```python
from build123d import *

# Parameters (mm, degrees)
PAD007_DEPTH          = 0.8
PAD007_MIRROR_2_DEPTH = 0.8


with BuildPart() as part:
    # Sketch038 (on XZ_Plane013 of Origin026) → Pad007 (new body, symmetric)
    with BuildSketch(Plane.XZ):
        with BuildLine():
            Line((0, 6.3), (0, 0))
            Line((0, 0), (-8.5, 0))
            ThreePointArc((-8.5, 0), (-10, 1.5), (-11.5, 0))
            Line((-11.5, 0), (-12.5, 0))
            ThreePointArc((-10, 2.5), (-11.767767, 1.767767), (-12.5, 0))
            Line((-10, 2.5), (-7.85, 2.5))
            Line((-7.85, 2.5), (-7.85, 6.3))
            Line((-7.85, 6.3), (0, 6.3))
        make_face()
    pad007 = extrude(amount=PAD007_DEPTH, both=True)

    # Sketch038 Mirror 2 → Pad007 Mirror 2 (add, symmetric)
    with BuildSketch(Plane(origin=(0, 0, 0), x_dir=(-1, 0, 0), z_dir=(0, 1, 0))):
        with BuildLine():
            Line((0, 6.3), (0, 0))
            Line((0, 0), (-8.5, 0))
            ThreePointArc((-8.5, 0), (-10, 1.5), (-11.5, 0))
            Line((-11.5, 0), (-12.5, 0))
            ThreePointArc((-10, 2.5), (-11.767767, 1.767767), (-12.5, 0))
            Line((-10, 2.5), (-7.85, 2.5))
            Line((-7.85, 2.5), (-7.85, 6.3))
            Line((-7.85, 6.3), (0, 6.3))
        make_face()
    pad007_mirror_2 = extrude(amount=-PAD007_MIRROR_2_DEPTH, both=True)

    # Mirror001: Pad007, Pad007 Mirror 2 across Sketch038 H_Axis
    add(pad007.mirror(Plane(origin=(0, 0, 0), x_dir=(0, -1, 0), z_dir=(0, 0, 1))))
    add(pad007_mirror_2.mirror(Plane(origin=(0, 0, 0), x_dir=(0, -1, 0), z_dir=(0, 0, 1))))


solid = part.part
```
Source: CAD feature listing. Evaluate the final solid. Frame: model axes, mm. A direction names the side the tool comes from. Coordinates: 2 decimals unless noted, no trailing zeros. Write each loop counter-clockwise with the first axis right and the second up, starting at its lowest first coordinate (ties: lowest second). Pieces come first, ordered by that corner, then holes. Notation, with made-up numbers: M 64.25,-29.5 L 89.25,-29.5 A31 cw 89.25,0.5 Z; hole C 21.25,-34.5 d8. An arc over 180 degrees is marked long. Answer as a JSON object with one key per item and string values.
1. Cut plane D-D on z = -4.75. Output: boundary loops of the cut face in (x, y).
Evaluation:
{"outline": "M -7.85,-0.8 L 7.85,-0.8 L 7.85,0.8 L -7.85,0.8 Z"}
2. Cut plane C-C on z = 2. Output: boundary loops of the cut face in (x, y), plus the area to 3 significant figures.
Evaluation:
{"outline": "M -11.5,-0.8 L 11.5,-0.8 L 11.5,0.8 L -11.5,0.8 Z", "area": "36.8 mm^2"}
3. Cut plane B-B on z = -0.5. Output: boundary loops of the cut face in (x, y), plus the area to 3 significant figures.
Evaluation:
{"outline": "M -12.45,-0.8 L -11.41,-0.8 L -11.41,0.8 L -12.45,0.8 Z; M -8.59,-0.8 L 8.59,-0.8 L 8.59,0.8 L -8.59,0.8 Z; M 11.41,-0.8 L 12.45,-0.8 L 12.45,0.8 L 11.41,0.8 Z", "area": "30.8 mm^2"}
4. Cut plane A-A on y = 0.45. Output: boundary loops of the cut face in (x, z), plus the area to 3 significant figures.
Evaluation:
{"outline": "M -10,-2.5 L -7.85,-2.5 L -7.85,-6.3 L 7.85,-6.3 L 7.85,-2.5 L 10,-2.5 A2.5 ccw 10,2.5 L 7.85,2.5 L 7.85,6.3 L -7.85,6.3 L -7.85,2.5 L -10,2.5 A2.5 ccw Z; hole C -10,0 d3; hole C 10,0 d3", "area": "225 mm^2"}
5. Ray query, L1, parallel to X at y = 0.2, z = 0; L2, parallel to X at y = -0.05, z = 0.5; L3, parallel to Z at x = 10, y = -0.05. Return the intervals inside material, ascending.
Evaluation:
{"L1": "-12.5 to -11.5, -8.5 to 8.5, 11.5 to 12.5", "L2": "-12.45 to -11.41, -8.59 to 8.59, 11.41 to 12.45", "L3": "-2.5 to -1.5, 1.5 to 2.5"}
6. Access query for faces 1 (the flat face through (-9, 0, -2.5)), 2 (the flat face through (7.85, 0, -4)), 3 (the flat face through (7.85, 0, 4)), 4 (the flat face through (-7.85, 0, 4)). Directions: +Z, -Z, +X, -X, +Y, -Y. A direction counts if a zero-diameter tool reaches every point of the face in a straight line with its end or side. Return the directions, or none.
Evaluation:
{"face 1": "-Z, -X, +Y, -Y", "face 2": "-Z, +X, +Y, -Y", "face 3": "+Z, +X, +Y, -Y", "face 4": "+Z, -X, +Y, -Y"}
7. Contact query for flat-ended pins moving along their axis: P1, Ø0.8, axis at x = 9, y = 0, coming from the -Z side; P2, Ø0.5, axis at y = 0, z = -4.5, coming from the -X side; P3, Ø0.8, axis at x = -8.5, y = 0, coming from the +Z side. Output: stop coordinate, or through.
Evaluation:
{"P1": "z = -2.5", "P2": "x = -7.85", "P3": "z = 2.5"}
8. Draft query along Z for faces 5 (the flat face through (-7.85, 0, -4)), 6 (the cylindrical face through (11.5, -0.01, -0.07)), 7 (the flat face through (9, 0, 2.5)). Return one class per face: released by +Z, released by -Z, zero draft, split by the parting line, or undercut.
Evaluation:
{"face 5": "zero draft", "face 6": "undercut", "face 7": "released by +Z"}
